For this review, take the finished solid that the model builds, in its own axes (mm). Face numbers are marked on the shaded views. Give positions to 0.01 mm unless a question says otherwise; leave off trailing zeros. Write each loop counter-clockwise with the first axis right and the second up, starting at its lowest first coordinate (ties: lowest second). Pieces come first, ordered by that corner, then holes.
1) We need section A-A on y = 0. Give the boundary of the cut face in (x, z), and give its area (3 significant figures).
2) Wall thickness on line 1 along Y through (x, z) = (0, -1.75); line 2 along Z through (x, y) = (-4.5, -3.75); line 3 along Y through (x, z) = (0, 0.75): over which ranges is each line inside the solid? List them lowest first.
3) Draft analysis for pull direction X (two halves, no side actions). For the marked faces 1, 2 and 3, state which applies: pulls with the +X half, pulls with the -X half, needs draft (parallel to the pull), parting line crosses it, or undercut.
4) We need section C-C on z = -0.5. Give the boundary of the cut face in (x, y), and give its area (3 significant figures).
5) For P1, Ø1.5, axis at y = 5, z = -1, coming from the -X side; P2, Ø3, axis at x = -3.5, z = 0, coming from the +Y side, all flat-tipped, find the tip position at first contact; note any pin that passes through.
6) We need section D-D on z = 0.75. Give the boundary of the cut face in (x, y), and give its area (3 significant figures).
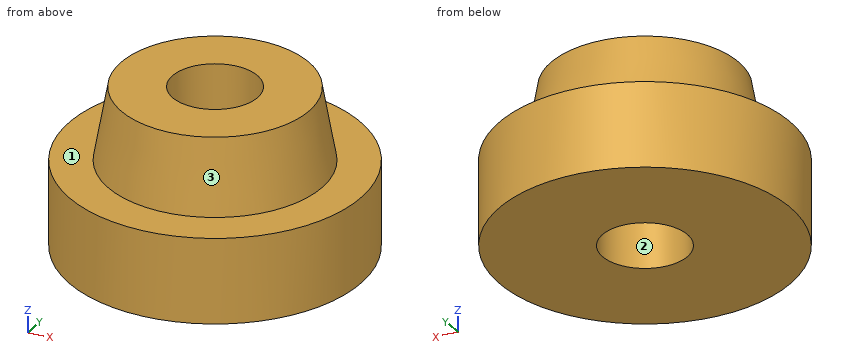
Autodesk Inventor part; units mm, degrees
ref_plane "YZ Plane" through (0, 0, 0) normal (1, 0, 0) x (0, 1, 0)
ref_plane "XZ Plane" through (0, 0, 0) normal (0, 1, 0) x (-1, 0, 0)
ref_plane "XY Plane" through (0, 0, 0) normal (0, 0, 1) x (1, 0, 0)
sketch "Sketch1" plane through (0, 0, 0) normal (0, 0, 1) x (1, 0, 0)
  circle A0 centre (0, 0) radius 6
  circle A1 centre (0, 0) radius 4.4
  dimension "d0" = 12
  dimension "d1" = 8.8
extrude "Extrusion1" add sketch "Sketch1" against normal blind 3.5 contours A0 | A1
extrude "Extrusion2" add sketch "Sketch1" along normal blind 3 draft -10 contours A1
hole "Hole1" at (0, 0, 3) direction (0, 0, -1) diameter 3.5 end through all
properties part number "segment0_coupler1" material "ABS Plastic"
Results list:
1. outline: (-6, -3.5) - (-1.75, -3.5) - (-1.75, 3) - (-3.87, 3) - (-4.4, 0) - (-6, 0) - close; (1.75, -3.5) - (6, -3.5) - (6, 0) - (4.4, 0) - (3.87, 3) - (1.75, 3) - close
1. area: 44.1 mm2
2. line 1: y = -6 to -1.75, 1.75 to 6
2. line 2: z = -3.5 to 0
2. line 3: y = -4.27 to -1.75, 1.75 to 4.27
3. face 1: needs draft
3. face 2: undercut
3. face 3: parting line crosses it
4. outline: circle Ø12 at (0, 0); hole circle Ø3.5 at (0, 0)
4. area: 103 mm2
5. P1: stops at x = -4.24
5. P2: stops at y = 5.66
6. outline: circle Ø8.54 at (0, 0); hole circle Ø3.5 at (0, 0)
6. area: 47.6 mm2
